The model under review builds one solid part; all positions refer to its coordinate system, in mm. Face numbers are marked on the shaded views. Give positions to 0.01 mm unless a question says otherwise; leave off trailing zeros. Order: outer loops, then holes, each group sorted by start corner. A loop starts at its lowest first (then second) coordinate and runs counter-clockwise, first axis right, second up. Notation, with made-up numbers: M 14,-36 L 65,-36 A17 cw 65,-13 Z; hole C -38.5,83 d3. An arc over 180 degrees is marked long. One line per question, with ' | ' between items. Start each with the question number.
1. Insertion check: P1, Ø1.5, axis at y = 4.5, z = 31, coming from the +X side; P2, Ø0.8, axis at x = 3.5, y = 8.5, coming from the +Z side; P3, Ø0.8, axis at y = 8.5, z = 8.5, coming from the -X side. Each pin has a flat end and moves straight along its axis. Give the tip position at first contact, or say it passes through.
2. The part is to be moulded in two halves that separate along Z. For the marked faces 1, 2 and 3, say which applies: +Z half, -Z half, draft (parallel to the pull), parting line (faces both ways), or undercut.
3. We need section A-A on x = 17.5. Write out the cut boundary in (y, z), then the cut area to 3 significant figures.
4. Wall thickness on L1, parallel to Z at x = 16, y = 7; L2, parallel to Y at x = 4.5, z = 34; L3, parallel to Y at x = 0.5, z = 44: over which ranges is each line inside the solid? List them lowest first.
5. We need section B-B on z = 43. Count the separate pieces of the cut face and the enclosed holes in it, then the cut area to 3 significant figures.
```python
from build123d import *

# Parameters (mm, degrees)
BOSS_EXTRUDE2_DEPTH      = 52
FILLET2_R                = 1
CUT_EXTRUDE2_DEPTH       = 3
CUT_EXTRUDE2_DEPTH_BACK  = 6
SKETCH10_W               = 2.350757351
SKETCH10_H               = 46
SKETCH11_W               = 17
SKETCH11_H               = 15
PELTIER_DEPTH            = 10
SKETCH12_W               = 21
SKETCH12_H               = 29
BATTERY_DEPTH            = 0.4
SKETCH14_W               = 21.3
SKETCH14_H               = 1
BOSS_EXTRUDE4_DEPTH      = 7.999920354
SKETCH15_W               = 3.297714658
SKETCH15_H               = 0.629450307
CUT_EXTRUDE5_DEPTH       = 3.6
SKETCH16_W               = 2.795507754
SKETCH16_H               = 0.669410668
CUT_EXTRUDE6_DEPTH       = 4.337027413
FILLET3_R                = 1
CUT_EXTRUDE7_DEPTH       = 1.6
CUT_EXTRUDE8_DEPTH       = 1.6
FILLET4_R                = 1
FILLET5_R                = 1
SKETCH19_W               = 21.3
SKETCH19_H               = 1
BOSS_EXTRUDE5_DEPTH      = 23.6
SKETCH20_W               = 7.625924169
SKETCH20_H               = 2.120993271
CUT_EXTRUDE9_DEPTH       = 2.6
SKETCH21_W               = 21.3
SKETCH21_H               = 2.886084762
BOSS_EXTRUDE6_DEPTH      = 8
SKETCH22_W               = 17
SKETCH22_H               = 1.5
BOSS_EXTRUDE7_DEPTH      = 22
SKETCH23_W               = 24.481547991
SKETCH23_H               = 2.403526745
CUT_EXTRUDE10_DEPTH      = 2
SKETCH24_W               = 15
SKETCH24_H               = 0.211445756
BOSS_EXTRUDE8_DEPTH      = 2
SKETCH25_W               = 4.787241237
SKETCH25_H               = 0.237383131
BOSS_EXTRUDE9_DEPTH      = 2
SKETCH26_W               = 11.036128308
SKETCH26_H               = 2.126226966
CUT_EXTRUDE11_DEPTH      = 2
CUT_EXTRUDE12_DEPTH      = 2
CUT_EXTRUDE12_DEPTH_BACK = 11
SKETCH27_W               = 46
SKETCH27_H               = 2.33
SKETCH28_W               = 1.978966
SKETCH28_H               = 14.822133623
SKETCH28_H_2             = 14.389327905
SKETCH28_W_2             = 1.978965999
CUT_EXTRUDE13_DEPTH      = 3


with BuildPart() as part:
    # Sketch1 → Boss-Extrude2 (new body)
    with BuildSketch(Plane.XY):
        with BuildLine():
            Line((-4.066957942, -1.190846618), (-7.240355005, -0.354620493))
            add(Edge.make_bspline(
                [(0.042333709, 8.998333002), (-4.213116867, 8.648828695), (-5.962383558, 1.81462105), (-7.240355005, -0.354620493)],
                knots=[0, 0, 0, 0, 1, 1, 1, 1], degree=3))
            Line((0.042333709, 8.998333002), (0.742333709, 8.998333002))
            Line((0.742333709, 8.998333002), (0.742333709, 1))
            Line((0.742333709, 1), (22.042333709, 1))
            Line((22.042333709, 1), (22.042333709, 8.998333002))
            Line((22.042333709, 8.998333002), (23.042333709, 8.998333002))
            add(Edge.make_bspline(
                [(23.042333709, 8.998333002), (27.852391375, 8.27132168), (31.467788923, -0.354620493)],
                knots=[0, 0, 0, 1, 1, 1], degree=2))
            Line((31.467788923, -0.354620493), (26.875523276, -1.190846618))
            add(Edge.make_bspline(
                [(22.86911945, 0), (24.564241842, 0.074416087), (25.297281614, 0.429058332), (26.875523276, -1.190846618)],
                knots=[0, 0, 0, 0, 1, 1, 1, 1], degree=3))
            Line((22.86911945, 0), (0, 0))
            add(Edge.make_bspline(
                [(0, 0), (-1.870814346, -0.163675047), (-2.239916233, 0.430706612), (-4.066957942, -1.190846618)],
                knots=[0, 0, 0, 0, 1, 1, 1, 1], degree=3))
        make_face()
    extrude(amount=BOSS_EXTRUDE2_DEPTH)

    # Fillet2
    fillet2_edges = [part.edges().sort_by_distance(p)[0] for p in [
        (-4.066957942, -1.190846618, 26),
        (-7.240355005, -0.354620493, 26),
    ]]
    fillet(fillet2_edges, radius=FILLET2_R)

    # Sketch10 → Cut-Extrude2 (cut, two sides: drawn at the far end of the back side and taken through both)
    with BuildSketch(Plane(origin=(-4.380890916, 3.569201652, 0), x_dir=(0.6316290075695021, 0.7752707893354205, 0), z_dir=(-0.7752707893354205, 0.6316290075695021, 0)).offset(-CUT_EXTRUDE2_DEPTH_BACK)):
        with Locations((-1.831509184, -27)):
            Rectangle(SKETCH10_W, SKETCH10_H)
    extrude(amount=CUT_EXTRUDE2_DEPTH + CUT_EXTRUDE2_DEPTH_BACK, mode=Mode.SUBTRACT)

    # Sketch11 → Peltier (cut)
    with BuildSketch(Plane(origin=(0, 1, 0), x_dir=(1, 0, 0), z_dir=(0, 1, 0))):
        with Locations((12.114692368, -9.5)):
            Rectangle(SKETCH11_W, SKETCH11_H)
    extrude(amount=-PELTIER_DEPTH, mode=Mode.SUBTRACT)

    # Sketch12 → Battery (cut)
    with BuildSketch(Plane(origin=(0, 1, 0), x_dir=(1, 0, 0), z_dir=(0, 1, 0))):
        with Locations((11.242333709, -36.5)):
            Rectangle(SKETCH12_W, SKETCH12_H)
    extrude(amount=-BATTERY_DEPTH, mode=Mode.SUBTRACT)

    # Sketch14 → Boss-Extrude4 (add)
    with BuildSketch(Plane(origin=(0, 1, 0), x_dir=(1, 0, 0), z_dir=(0, 1, 0))):
        with Locations((11.392333709, -51.5)):
            Rectangle(SKETCH14_W, SKETCH14_H)
    extrude(amount=BOSS_EXTRUDE4_DEPTH)

    # Sketch15 → Cut-Extrude5 (cut)
    with BuildSketch(Plane(origin=(3.614692368, 0, 0), x_dir=(0, 0, -1), z_dir=(1, 0, 0))):
        with Locations((-15.351142671, 0.685274847)):
            Rectangle(SKETCH15_W, SKETCH15_H)
    extrude(amount=-CUT_EXTRUDE5_DEPTH, mode=Mode.SUBTRACT)

    # Sketch16 → Cut-Extrude6 (cut)
    with BuildSketch(Plane(origin=(3.614692368, 0, 0), x_dir=(0, 0, -1), z_dir=(1, 0, 0))):
        with Locations((-2.862635658, 0.665294666)):
            Rectangle(SKETCH16_W, SKETCH16_H)
    extrude(amount=-CUT_EXTRUDE6_DEPTH, mode=Mode.SUBTRACT)

    # Fillet3
    # the kernel refuses this fillet: 1 mm, written as the material it takes off along each edge
    with BuildSketch(Plane(origin=(3.614692368, 0.330589332, 2), x_dir=(0, -1, 0), z_dir=(0, 0, 1))) as fillet3_piece_1:
        with BuildLine():
            CenterArc((1, -0.742892561), FILLET3_R, 132.021596152, 47.978403848)
            Line((0, -0.742892561), (0, 0))
            Line((0, 0), (0.330589332, 0))
        make_face()
    extrude(amount=2.260389535, mode=Mode.SUBTRACT)
    with BuildSketch(Plane(origin=(3.614692368, 0.370549693, 17), x_dir=(0, -1, 0), z_dir=(0, 0, -1))) as fillet3_piece_2:
        with BuildLine():
            CenterArc((1, 0.77704074), FILLET3_R, 180, 50.990421184)
            Line((0, 0.77704074), (0, 0))
            Line((0, 0), (0.370549693, 0))
        make_face()
    extrude(amount=3.297714658, mode=Mode.SUBTRACT)

    # Sketch17 → Cut-Extrude7 (cut)
    with BuildSketch(Plane(origin=(0.742333709, 0, 0), x_dir=(0, 0, -1), z_dir=(1, 0, 0))):
        with BuildLine():
            Line((-26.679947222, 8.607264172), (-26.679947222, 5.897267678))
            add(Edge.make_bspline(
                [(-4.260389535, 1), (-14.867625221, 6.272509714), (-26.679947222, 5.897267678)],
                knots=[0, 0, 0, 1, 1, 1], degree=2))
            Line((-4.260389535, 1), (-1.464881781, 1))
            add(Edge.make_bspline(
                [(-1.464881781, 1), (-12.835212302, 8.374655541), (-26.679947222, 8.607264172)],
                knots=[0, 0, 0, 1, 1, 1], degree=2))
        make_face()
    extrude(amount=-CUT_EXTRUDE7_DEPTH, mode=Mode.SUBTRACT)

    # Sketch18 → Cut-Extrude8 (cut)
    with BuildSketch(Plane(origin=(0.742333709, 0, 0), x_dir=(0, 0, -1), z_dir=(1, 0, 0))):
        with BuildLine():
            Line((-27.127269804, 2.333242891), (-27.127269804, 5.881050361))
            add(Edge.make_bspline(
                [(-13.702285342, 1), (-19.59820355, 6.798459793), (-27.127269804, 5.881050361)],
                knots=[0, 0, 0, 1, 1, 1], degree=2))
            Line((-13.702285342, 1), (-17, 1))
            add(Edge.make_bspline(
                [(-17, 1), (-21.902562333, 3.381704282), (-27.127269804, 2.333242891)],
                knots=[0, 0, 0, 1, 1, 1], degree=2))
        make_face()
    extrude(amount=-CUT_EXTRUDE8_DEPTH, mode=Mode.SUBTRACT)

    # Fillet4
    fillet4_edges = [part.edges().sort_by_distance(p)[0] for p in [
        (26.875523276, -1.190846618, 26),
    ]]
    fillet(fillet4_edges, radius=FILLET4_R)

    # Fillet5
    fillet5_edges = [part.edges().sort_by_distance(p)[0] for p in [
        (31.467788923, -0.354620493, 26),
    ]]
    fillet(fillet5_edges, radius=FILLET5_R)

    # Sketch19 → Boss-Extrude5 (add)
    with BuildSketch(Plane(origin=(0, 0, 51), x_dir=(-1, 0, 0), z_dir=(0, 0, -1))):
        with Locations((-11.392333709, 5)):
            Rectangle(SKETCH19_W, SKETCH19_H)
    extrude(amount=BOSS_EXTRUDE5_DEPTH)

    # Sketch20 → Cut-Extrude9 (cut)
    with BuildSketch(Plane(origin=(0, 5.5, 0), x_dir=(1, 0, 0), z_dir=(0, 1, 0))):
        with Locations((11.936871332, -49.939503364)):
            Rectangle(SKETCH20_W, SKETCH20_H)
    extrude(amount=-CUT_EXTRUDE9_DEPTH, mode=Mode.SUBTRACT)

    # Sketch21 → Boss-Extrude6 (add)
    with BuildSketch(Plane(origin=(0, 1, 0), x_dir=(1, 0, 0), z_dir=(0, 1, 0))):
        with Locations((11.392333709, -18.443042381)):
            Rectangle(SKETCH21_W, SKETCH21_H)
    extrude(amount=BOSS_EXTRUDE6_DEPTH)

    # Sketch22 → Boss-Extrude7 (add)
    with BuildSketch(Plane.ZY.offset(-22.042333709)):
        with Locations((8.5, 8.25)):
            Rectangle(SKETCH22_W, SKETCH22_H)
    extrude(amount=BOSS_EXTRUDE7_DEPTH)

    # Sketch23 → Cut-Extrude10 (cut)
    with BuildSketch(Plane(origin=(0.742333709, 0, 0), x_dir=(0, 0, -1), z_dir=(1, 0, 0))):
        with Locations((-32.126858758, 6.701763373)):
            Rectangle(SKETCH23_W, SKETCH23_H)
    extrude(amount=-CUT_EXTRUDE10_DEPTH, mode=Mode.SUBTRACT)

    # Sketch24 → Boss-Extrude8 (add)
    with BuildSketch(Plane.ZY.offset(-20.614692368)):
        with Locations((9.5, 0.105722878)):
            Rectangle(SKETCH24_W, SKETCH24_H)
    extrude(amount=BOSS_EXTRUDE8_DEPTH)

    # Sketch25 → Boss-Extrude9 (add)
    with BuildSketch(Plane(origin=(3.614692368, 0, 0), x_dir=(0, 0, -1), z_dir=(1, 0, 0))):
        with Locations((-9.281203123, 0.118691566)):
            Rectangle(SKETCH25_W, SKETCH25_H)
    extrude(amount=BOSS_EXTRUDE9_DEPTH)

    # Sketch26 → Cut-Extrude11 (cut)
    with BuildSketch(Plane(origin=(0, 0, 51), x_dir=(-1, 0, 0), z_dir=(0, 0, -1))):
        with Locations((-6.260397863, 7.936806871)):
            Rectangle(SKETCH26_W, SKETCH26_H)
    extrude(amount=-CUT_EXTRUDE11_DEPTH, mode=Mode.SUBTRACT)

    # Sketch27 → Cut-Extrude12 (cut, two sides: drawn at the far end of the back side and taken through both)
    with BuildSketch(Plane(origin=(16.401330443, 15.864191281, 0), x_dir=(0, 0, -1), z_dir=(0.7187787233935903, 0.6952389134654942, 0)).offset(-CUT_EXTRUDE12_DEPTH_BACK)):
        with Locations((-26, -18.013212029)):
            Rectangle(SKETCH27_W, SKETCH27_H)
    extrude(amount=CUT_EXTRUDE12_DEPTH + CUT_EXTRUDE12_DEPTH_BACK, mode=Mode.SUBTRACT)

    # Sketch28 → Cut-Extrude13 (cut)
    with BuildSketch(Plane(origin=(0, 9, 0), x_dir=(1, 0, 0), z_dir=(0, 1, 0))):
        with Locations((19.299375066, -8.918059871)):
            Rectangle(SKETCH28_W, SKETCH28_H)
        with Locations((15.520409066, -9.13446273)):
            Rectangle(SKETCH28_W, SKETCH28_H_2)
        with Locations((11.741443067, -8.918059871)):
            Rectangle(SKETCH28_W_2, SKETCH28_H)
        with Locations((7.962477067, -8.918059871)):
            Rectangle(SKETCH28_W, SKETCH28_H)
        with Locations((4.183511067, -8.918059871)):
            Rectangle(SKETCH28_W, SKETCH28_H)
    extrude(amount=-CUT_EXTRUDE13_DEPTH, mode=Mode.SUBTRACT)


solid = part.part
```
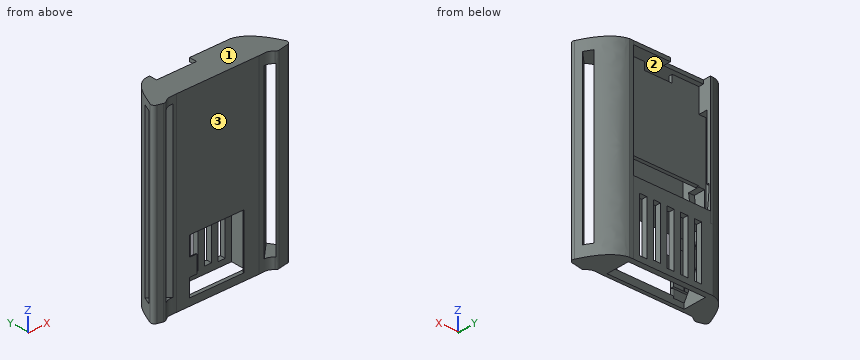
Entries:
1) P1: stops at x = 28.92 | P2: stops at z = 19.89 | P3: stops at x = -2.23
2) face 1: +Z half | face 2: undercut | face 3: draft
3) outline: M 0,0 L 1,0 L 1,2 L 0,2 Z; M 0,17 L 7.5,17 L 7.5,0 L 9,0 L 9,19.89 L 1,19.89 L 1,22 L 0.6,22 L 0.6,51 L 4.5,51 L 4.5,27.4 L 5.5,27.4 L 5.5,51 L 9,51 L 9,52 L 0,52 Z | area: 106 mm^2
4) L1: z = 17 to 19.89, 51 to 52 | L2: y = 0 to 0.6, 4.5 to 5.5 | L3: y = 0 to 5.5, 7.9 to 9
5) separate pieces: 3 | enclosed holes: 1 | area: 120 mm^2
